Can you work these out from the model? Positions are in its coordinate system, mm. Face numbers are marked on the shaded views. A direction names the side the tool comes from. Give positions to 0.01 mm unless a question says otherwise; leave off trailing zeros. Loops run counter-clockwise (first coordinate to the right, second up) from the corner with the lowest first, then second, coordinate; pieces in that order, holes last.
from build123d import *

# Parameters (mm, degrees)
F1_DEPTH = 7


with BuildPart() as f1:
    # F0 (on Top) → F1 (new body)
    with BuildSketch(Plane.XY):
        with BuildLine():
            ThreePointArc((-3.952456, 0.032943), (-2.452339, 0.027193), (-0.952456, 0))
            Line((-0.952456, 0), (-0.952456, 2.2))
            Line((-0.952456, 2.2), (0.247544, 3))
            Line((0.247544, 3), (-3.152456, 7.348705))
            Line((-3.152456, 7.348705), (-3.952456, 7.348705))
            Line((-3.952456, 7.348705), (-3.952456, 2.5))
            Line((-3.952456, 2.5), (-3.952456, 2.388958))
            ThreePointArc((-3.952456, 2.388958), (-12.602156, 1.550858), (-21.152861, 0))
            Line((-21.152861, 0), (-20.925339, -1.405665))
            ThreePointArc((-20.925339, -1.405665), (-12.468133, -0.341437), (-3.952456, 0.032943))
        make_face()
    extrude(amount=F1_DEPTH)


solid = f1.part
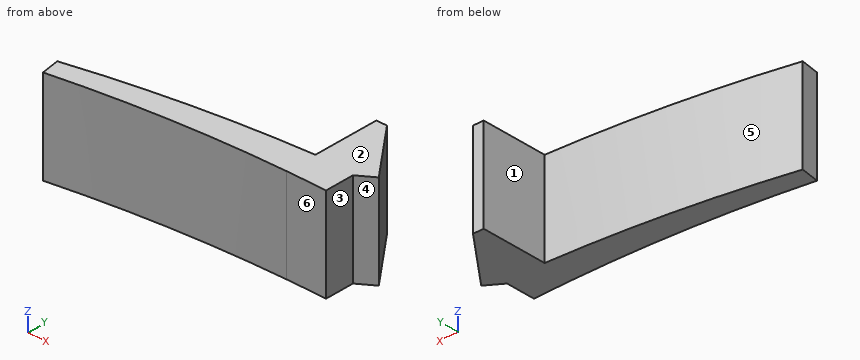
(1) Will these pins go through, and if not, where does the flat tip stop? P1, Ø2.5, axis at y = 1.5, z = 2.5, coming from the +X side; P2, Ø2, axis at y = 3.5, z = 4, coming from the -X side.
Returned:
P1: stops at x = -0.13
P2: stops at x = -3.95
(2) Which directions (+Z, -Z, +X, -X, +Y, -Y) give clear straight access to the entire face, cutting with the end or side of a thin tool? Please do the marked faces 1, 2 and 3.
Returned:
face 1: +Z, -Z, -X, +Y
face 2: +Z, +X, -X, +Y, -Y
face 3: +Z, -Z, +X, -Y
(3) Suppose I cut it at B-B on x = -10.5. List the corners of the cut face in (y, z) for me, plus the area to 3 significant figures.
Returned:
outline: (-0.19, 0) - (1.82, 0) - (1.82, 7) - (-0.19, 7) - close
area: 14.1 mm2
(4) Suppose I cut it at C-C on y = -0.5. List the corners of the cut face in (x, z) for me, plus the area to 3 significant figures.
Returned:
outline: (-21.07, 0) - (-14.17, 0) - (-14.17, 7) - (-21.07, 7) - close
area: 48.3 mm2
(5) Please list where these lines run through material, in increasing order: probe 1 along Y at (x, z) = (-4, 1.75); probe 2 along Y at (x, z) = (-3.25, 1.5); probe 3 along X at (y, z) = (7, 5.5).
Returned:
probe 1: y = 0.03 to 2.39
probe 2: y = 0.03 to 7.35
probe 3: x = -3.95 to -2.88
(6) Thinking about a two-plate mould opening in X: for the marked faces 4, 5 and 6, which applies, pulls with the +X half, pulls with the -X half, needs draft (parallel to the pull), parting line crosses it, or undercut?
Returned:
face 4: pulls with the +X half
face 5: pulls with the -X half
face 6: undercut
(7) Suppose I cut it at A-A on z = 6.5. List the corners of the cut face in (x, y) for me.
Returned:
outline: (-21.15, 0) - (-20.93, -1.41) arc R104.95 cw to (-3.95, 0.03) arc R104.94 cw to (-0.95, 0) - (-0.95, 2.2) - (0.25, 3) - (-3.15, 7.35) - (-3.95, 7.35) - (-3.95, 2.39) arc R104.95 ccw to start
